Print and shaded views of the part. All mm, measured from the part's lowest x, y and z. Coordinates: 2 decimals unless noted, no trailing zeros. Loops run counter-clockwise (first coordinate to the right, second up) from the corner with the lowest first, then second, coordinate; pieces in that order, holes last. Notation, with made-up numbers: M 80,-31 L 88,-31 A24 cw 88,-20 Z; hole C 83.5,29 d4. An arc over 180 degrees is marked long. Use a Markdown table: item, result. Add a question column.
1) Band-saw the part on C-C (z = 9.5). List the corners of the cut face in (x, y), plus the area to 3 significant figures.
2) Wall check: probe 1 along X at (y, z) = (13, 8.5); probe 2 along X at (y, z) = (8, 15.5); probe 3 along Z at (x, y) = (43.5, 33.5). Give the ranges that are in metal, low to high. Write a range as from..to.
3) Band-saw the part on A-A (y = 18.5). List the corners of the cut face in (x, z).
4) Pin check, flat tips, straight feed: pin 1 Ø2 at (x, y) = (33, 38.5) entering from -Z; pin 2 Ø1 at (x, y) = (33.5, 22.5) entering from -Z. Stop position of each tip, or through.
5) Band-saw the part on B-B (x = 43.5). List the corners of the cut face in (y, z), plus the area to 3 significant figures.
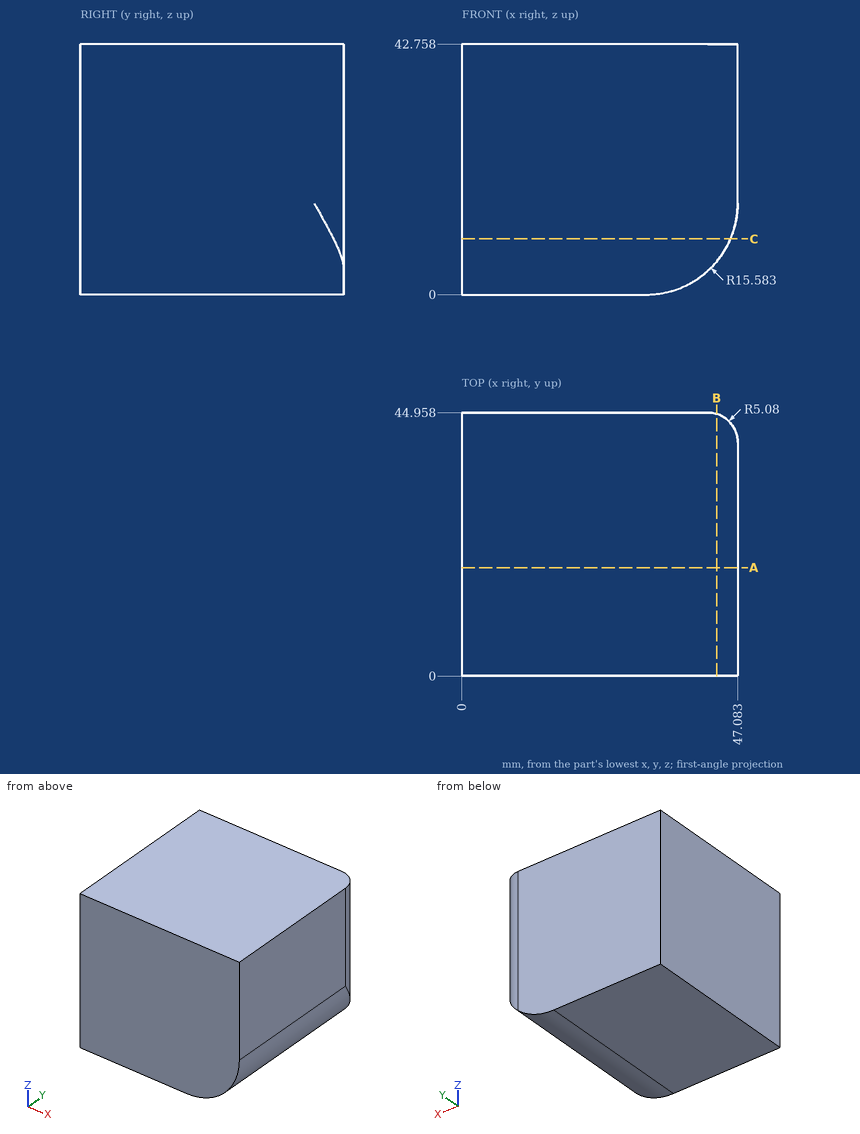
Entries:
| question | item | result |
|---|---|---|
| 1 | outline | M 0,0 L 45.85,0 L 45.85,43.2 A5.08 ccw 42,44.96 L 0,44.96 Z |
| 1 | area | 2,060 mm2 |
| 2 | probe 1 | 0..45.38 |
| 2 | probe 2 | 0..47.08 |
| 2 | probe 3 | 5.64..42.76 |
| 3 | outline | M 0,0 L 31.5,0 A15.58 ccw 47.08,15.58 L 47.08,42.76 L 0,42.76 Z |
| 4 | pin 1 | z = 0.01 |
| 4 | pin 2 | z = 0.07 |
| 5 | outline | M 0,5.64 L 44.73,5.64 L 44.73,42.76 L 0,42.76 Z |
| 5 | area | 1,660 mm2 |
